Read the model definition and answer for the solid it produces. Units are mm, in the model's axes. Face numbers are marked on the shaded views. A direction names the side the tool comes from. Give positions to 0.01 mm unless a question says otherwise; leave off trailing zeros. Loops run counter-clockwise (first coordinate to the right, second up) from the corner with the lowest first, then second, coordinate; pieces in that order, holes last. Notation, with made-up numbers: (37, 85.25) - (87, 85.25) arc R26 ccw to (87, 120.25) - close; hole circle Ø5 at (18, 47). An arc over 180 degrees is marked (long way). Use a Markdown table: item, result. Add a question column.
Item 1: For a pull along Z with two mould halves and no side action, classify the marked faces 1, 2 and 3 as +Z half, -Z half, draft (parallel to the pull), parting line (faces both ways), or undercut.
Item 2: A cutting plane is placed at C-C (y = -6.5). Determine the outline of the cut face in (x, z), plus the area to 3 significant figures.
Item 3: Consider probe 1 along Z at (x, y) = (0, -8.5); probe 2 along Y at (x, z) = (2.25, -2.25); probe 3 along Y at (x, z) = (1, 1.25). Determine where each line is inside the solid, lowest interval first. Write a range as [from, to].
Item 4: Which of the six approach directions +Z, -Z, +X, -X, +Y, -Y give full straight-line access (tool end or side, diameter ignored) to the marked faces 4, 5 and 6?
Item 5: Each of these flat-tipped pins is pushed along its axis until it touches: P1, Ø5, axis at x = -0.5, y = -11, coming from the +Z side; P2, Ø5, axis at x = 3, y = 1, coming from the +Z side; P3, Ø5, axis at y = -10, z = 0, coming from the +X side. Where does it stop, or does it pass through?
Item 6: A cutting plane is placed at A-A (x = 0). Determine the outline of the cut face in (y, z), plus the area to 3 significant figures.
Item 7: A cutting plane is placed at B-B (y = 1.5). Determine the outline of the cut face in (x, z).
Autodesk Inventor part; units mm, degrees
ref_plane "YZ Plane" through (0, 0, 0) normal (1, 0, 0) x (0, 1, 0)
ref_plane "XZ Plane" through (0, 0, 0) normal (0, 1, 0) x (-1, 0, 0)
ref_plane "XY Plane" through (0, 0, 0) normal (0, 0, 1) x (1, 0, 0)
sketch "Cap Cross Section" plane through (0, 0, 0) normal (0, 1, 0) x (-1, 0, 0)
  circle A0 centre (0, 0) radius 4.25
  dimension "d0" = 8.5
extrude "Cap" add sketch "Cap Cross Section" along normal blind 5
sketch "Key Socket Cutout Outline" plane through (0, 5, 0) normal (0, 1, 0) x (1, 0, 0)
  line L0 (1.1547, 2) -> (2.3094, 0)
  line L1 (2.3094, 0) -> (1.1547, -2)
  line L2 (1.1547, -2) -> (-1.1547, -2)
  line L3 (-1.1547, -2) -> (-2.3094, 0)
  line L4 (-2.3094, 0) -> (-1.1547, 2)
  line L5 (-1.1547, 2) -> (1.1547, 2)
  point P0 (0, 0)
  point P1 (0, 0)
  dimension "d3" = 4
extrude "Key Socket Cutout" cut sketch "Key Socket Cutout Outline" against normal blind 2.5
sketch "Body Cross Section" plane through (0, 0, 0) normal (0, -1, 0) x (1, 0, 0)
  circle A0 centre (0, 0) radius 2.5
  dimension "d6" = 5
extrude "Body" add sketch "Body Cross Section" along normal blind 20
thread "Thread"
fillet "Cap Fillet" radius 0.5 1 edges at (4.25, 5, 0)
properties part number "SSCF-M5-20-A4" material "Stainless Steel AISI 317"
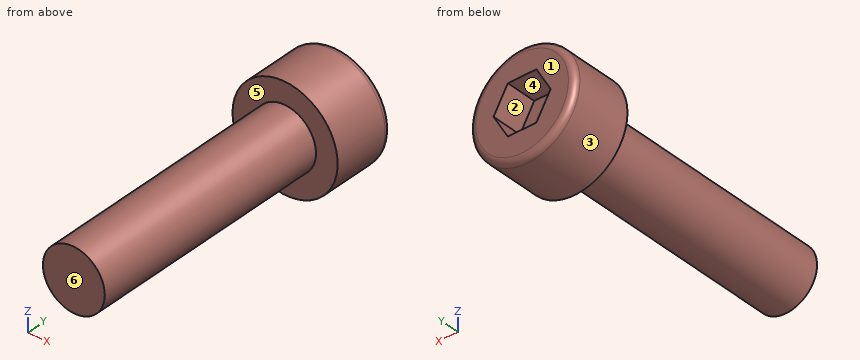
Geometry says:
| question | item | result |
|---|---|---|
| 1 | face 1 | draft |
| 1 | face 2 | undercut |
| 1 | face 3 | parting line |
| 2 | outline | circle Ø5 at (0, 0) |
| 2 | area | 19.6 mm² |
| 3 | probe 1 | [-2.5, 2.5] |
| 3 | probe 2 | [0, 5] |
| 3 | probe 3 | [-20, 2.5] |
| 4 | face 4 | +Y |
| 4 | face 5 | -Y |
| 4 | face 6 | +Z, -Z, +X, -X, -Y |
| 5 | P1 | z = 2.5 |
| 5 | P2 | z = 4.22 |
| 5 | P3 | x = 2.5 |
| 6 | outline | (-20, -2.5) - (0, -2.5) - (0, -4.25) - (4.5, -4.25) arc R0.5 ccw to (5, -3.75) - (5, -2) - (2.5, -2) - (2.5, 2) - (5, 2) - (5, 3.75) arc R0.5 ccw to (4.5, 4.25) - (0, 4.25) - (0, 2.5) - (-20, 2.5) - close |
| 6 | area | 132 mm² |
| 7 | outline | circle Ø8.5 at (0, 0) |
